Here's how the part is built. I have some questions about the finished solid (model axes, mm). Face numbers are marked on the shaded views. A direction names the side the tool comes from. Round coordinates to 2 decimals unless told otherwise and drop trailing zeros. Write each loop counter-clockwise with the first axis right and the second up, starting at its lowest first coordinate (ties: lowest second). Pieces come first, ordered by that corner, then holes. Notation, with made-up numbers: M -15,-8.75 L -5,-8.75 A27 cw -5,17.25 Z; hole C -1.75,0.5 d4. An arc over 180 degrees is marked long. Write item = value, one per line. Start each with the question number.
(1) I want a section at C-C (x = 47). List the corners of the cut face in (y, z) for me (3 decimals).
(2) I want a section at B-B (z = 30). Give the number of separate pieces and of enclosed holes in the cut face, and give its area (3 significant figures).
(3) On a 3-axis mill with a long thin cutter (end or side, diameter ignored), from which of +Z, -Z, +X, -X, +Y, -Y can I reach the whole of each face in a straight line? I mean the marked faces 4 and 5. Say none if no direction works.
(4) If we mould it in two halves opening along X, with no side actions, what happens to the marked faces 1, 2 and 3? For each: released by +X, released by -X, zero draft, split by the parting line, or undercut.
(5) Will these pins go through, and if not, where does the flat tip stop? pin 1 Ø3 at (x, z) = (58, 48) entering from +Y; pin 2 Ø1.8 at (x, z) = (35, 43) entering from -Y.
(6) I need wall thicknesses on line 1 along Z through (x, y) = (35, 7.5) (3 decimals); line 2 along X through (y, z) = (0.75, 30); line 3 along X through (y, z) = (16.5, 54). Which ranges of each line are inside material? Lowest first, please.
(7) I want a section at D-D (x = 35). List the corners of the cut face in (y, z) for me (3 decimals).
(8) I want a section at A-A (z = 18). List the corners of the cut face in (x, y) for me (3 decimals).
```python
from build123d import *

# Parameters (mm, degrees)
SKETCH3_W           = 70
SKETCH3_H           = 60
BOSS_EXTRUDE3_DEPTH = 20
SKETCH4_R           = 1.575
CUT_EXTRUDE1_DEPTH  = 95.339811321
SKETCH6_R           = 2.1
CUT_EXTRUDE2_DEPTH  = 95.339811321
SKETCH9_R           = 3.25
CUT_EXTRUDE3_DEPTH  = 95.339811321
CUT_EXTRUDE4_START  = -3
SKETCH11_R          = 3
SKETCH11_R_2        = 1.575
CUT_EXTRUDE4_DEPTH  = 3
CHAMFER1_SIZE       = 0.8
SKETCH12_R          = 5.05
CUT_EXTRUDE5_DEPTH  = 5


with BuildPart() as part:
    # Sketch3 → Boss-Extrude3 (new body)
    with BuildSketch(Plane(origin=(0, 0, 0), x_dir=(1, 0, 0), z_dir=(0, 1, 0))):
        with Locations((35, -30)):
            Rectangle(SKETCH3_W, SKETCH3_H)
    extrude(amount=BOSS_EXTRUDE3_DEPTH)

    # Sketch4 → Cut-Extrude1 (cut, through all)
    with BuildSketch(Plane(origin=(0, 20, 0), x_dir=(1, 0, 0), z_dir=(0, 1, 0))):
        with Locations(Location((35, -30, 0), (0, 0, 270))):
            Circle(SKETCH4_R)
        with Locations(Location((35, -18, 0), (0, 0, 270))):
            Circle(SKETCH4_R)
        with Locations(Location((47, -30, 0), (0, 0, 270))):
            Circle(SKETCH4_R)
        with Locations(Location((35, -42, 0), (0, 0, 270))):
            Circle(SKETCH4_R)
        with Locations(Location((23, -30, 0), (0, 0, 270))):
            Circle(SKETCH4_R)
    extrude(amount=-CUT_EXTRUDE1_DEPTH, mode=Mode.SUBTRACT)

    # Sketch6 → Cut-Extrude2 (cut, through all)
    with BuildSketch(Plane.XZ):
        with Locations(Location((59.875, 21.875, 0), (0, 0, 270))):
            Circle(SKETCH6_R)
        with Locations(Location((25.625, 21.875, 0), (0, 0, 270))):
            Circle(SKETCH6_R)
    extrude(amount=-CUT_EXTRUDE2_DEPTH, mode=Mode.SUBTRACT)

    # Sketch9 → Cut-Extrude3 (cut, through all)
    with BuildSketch(Plane(origin=(0, 0, 0), x_dir=(-1, 0, 0), z_dir=(0, 0, -1))):
        with Locations((-52.525, 10)):
            Circle(SKETCH9_R)
        with Locations((-16.175, 10)):
            Circle(SKETCH9_R)
    extrude(amount=-CUT_EXTRUDE3_DEPTH, mode=Mode.SUBTRACT)

    # Sketch11 → Cut-Extrude4 (cut)
    # profile 1 of 10: a face of its own
    with BuildSketch(Plane.XZ.offset(CUT_EXTRUDE4_START)):
        with Locations(Location((35, 18, 0), (0, 0, 270))):
            Circle(SKETCH11_R)
        with Locations(Location((35, 18, 0), (0, 0, 90))):
            Circle(SKETCH11_R_2, mode=Mode.SUBTRACT)
    # profile 2 of 10: a face of its own
    with BuildSketch(Plane.XZ.offset(CUT_EXTRUDE4_START)):
        with Locations(Location((35, 30, 0), (0, 0, 270))):
            Circle(SKETCH11_R)
        with Locations(Location((35, 30, 0), (0, 0, 90))):
            Circle(SKETCH11_R_2, mode=Mode.SUBTRACT)
    # profile 3 of 10: a face of its own
    with BuildSketch(Plane.XZ.offset(CUT_EXTRUDE4_START)):
        with Locations(Location((47, 30, 0), (0, 0, 270))):
            Circle(SKETCH11_R)
        with Locations(Location((47, 30, 0), (0, 0, 90))):
            Circle(SKETCH11_R_2, mode=Mode.SUBTRACT)
    # profile 4 of 10: a face of its own
    with BuildSketch(Plane.XZ.offset(CUT_EXTRUDE4_START)):
        with Locations(Location((23, 30, 0), (0, 0, 270))):
            Circle(SKETCH11_R)
        with Locations(Location((23, 30, 0), (0, 0, 90))):
            Circle(SKETCH11_R_2, mode=Mode.SUBTRACT)
    # profile 5 of 10: a face of its own
    with BuildSketch(Plane.XZ.offset(CUT_EXTRUDE4_START)):
        with Locations(Location((35, 42, 0), (0, 0, 270))):
            Circle(SKETCH11_R)
        with Locations(Location((35, 42, 0), (0, 0, 90))):
            Circle(SKETCH11_R_2, mode=Mode.SUBTRACT)
    # profile 6 of 10: a face of its own
    with BuildSketch(Plane.XZ.offset(CUT_EXTRUDE4_START)):
        with Locations(Location((35, 42, 0), (0, 0, 90))):
            Circle(SKETCH11_R_2)
    # profile 7 of 10: a face of its own
    with BuildSketch(Plane.XZ.offset(CUT_EXTRUDE4_START)):
        with Locations(Location((23, 30, 0), (0, 0, 90))):
            Circle(SKETCH11_R_2)
    # profile 8 of 10: a face of its own
    with BuildSketch(Plane.XZ.offset(CUT_EXTRUDE4_START)):
        with Locations(Location((35, 30, 0), (0, 0, 90))):
            Circle(SKETCH11_R_2)
    # profile 9 of 10: a face of its own
    with BuildSketch(Plane.XZ.offset(CUT_EXTRUDE4_START)):
        with Locations(Location((47, 30, 0), (0, 0, 90))):
            Circle(SKETCH11_R_2)
    # profile 10 of 10: a face of its own
    with BuildSketch(Plane.XZ.offset(CUT_EXTRUDE4_START)):
        with Locations(Location((35, 18, 0), (0, 0, 90))):
            Circle(SKETCH11_R_2)
    extrude(amount=CUT_EXTRUDE4_DEPTH, mode=Mode.SUBTRACT)

    # Chamfer1
    chamfer1_edges = [part.edges().sort_by_distance(p)[0] for p in [
        (55.775, 10, 0),
        (19.425, 10, 0),
    ]]
    chamfer(chamfer1_edges, length=CHAMFER1_SIZE)

    # Sketch12 → Cut-Extrude5 (cut)
    with BuildSketch(Plane(origin=(0, 20, 0), x_dir=(1, 0, 0), z_dir=(0, 1, 0))):
        with Locations((14.5, 0.104949747)):
            Circle(SKETCH12_R)
        with Locations((55.5, 0.104949747)):
            Circle(SKETCH12_R)
        with BuildLine():
            Line((9.45, -60.104949747), (9.45, -44.5))
            ThreePointArc((9.45, -44.5), (14.5, -39.45), (19.55, -44.5))
            Line((19.55, -44.5), (19.55, -60.104949747))
            ThreePointArc((19.55, -60.104949747), (14.5, -65.154949747), (9.45, -60.104949747))
        make_face()
        with BuildLine():
            Line((60.55, -60.104949747), (60.55, -44.5))
            ThreePointArc((60.55, -44.5), (55.5, -39.45), (50.45, -44.5))
            Line((50.45, -44.5), (50.45, -60.104949747))
            ThreePointArc((50.45, -60.104949747), (55.5, -65.154949747), (60.55, -60.104949747))
        make_face()
    extrude(amount=-CUT_EXTRUDE5_DEPTH, mode=Mode.SUBTRACT)


solid = part.part
```
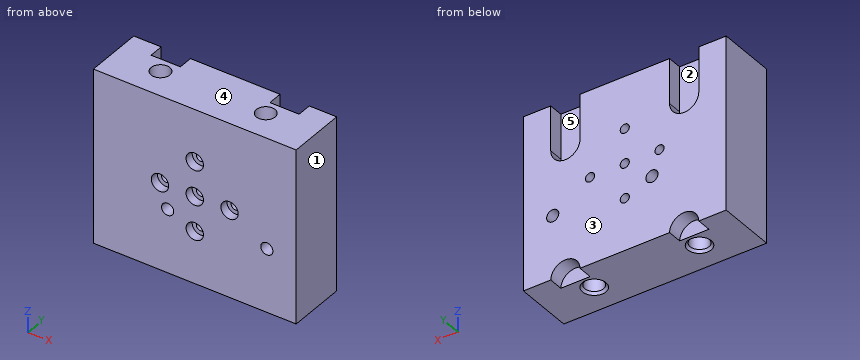
Returned:
q1.outline = M 0,0 L 20,0 L 20,28.425 L 3,28.425 L 3,27 L 0,27 Z; M 0,33 L 3,33 L 3,31.575 L 20,31.575 L 20,60 L 0,60 Z
q2.separate_pieces = 4
q2.enclosed_holes = 2
q2.area = 1,120 mm²
q3.face_4 = +Z, +X, -X, +Y, -Y
q3.face_5 = +Z, +Y
q4.face_1 = released by +X
q4.face_2 = undercut
q4.face_3 = zero draft
q5.pin_1 = 15
q5.pin_2 = 3
q6.line_1 = 0 to 16.425, 19.575 to 28.425, 31.575 to 40.425, 43.575 to 60
q6.line_2 = 0 to 20, 26 to 32, 38 to 44, 50 to 70
q6.line_3 = 0 to 9.45, 19.55 to 50.45, 60.55 to 70
q7.outline = M 0,0 L 20,0 L 20,16.425 L 3,16.425 L 3,15 L 0,15 Z; M 0,21 L 3,21 L 3,19.575 L 20,19.575 L 20,28.425 L 3,28.425 L 3,27 L 0,27 Z; M 0,33 L 3,33 L 3,31.575 L 20,31.575 L 20,40.425 L 3,40.425 L 3,39 L 0,39 Z; M 0,45 L 3,45 L 3,43.575 L 20,43.575 L 20,60 L 0,60 Z
q8.outline = M 0,0 L 32,0 L 32,3 L 33.425,3 L 33.425,20 L 0,20 Z; M 36.575,3 L 38,3 L 38,0 L 70,0 L 70,20 L 36.575,20 Z; hole C 16.175,10 d6.5; hole C 52.525,10 d6.5
